from build123d import *

# Parameters (mm, degrees)
BOSS_EXTRUDE1_DEPTH = 4


with BuildPart() as part:
    # Sketch1 → Boss-Extrude1 (new body)
    with BuildSketch(Plane(origin=(0, 0, 0), x_dir=(1, 0, 0), z_dir=(0, 1, 0))):
        with BuildLine():
            ThreePointArc((-5.5, 7.415063509), (-5.646446609, 7.7686169), (-6, 7.915063509))
            Line((-6, 7.915063509), (-9, 7.915063509))
            ThreePointArc((-9, 7.915063509), (-9.353553391, 7.7686169), (-9.5, 7.415063509))
            Line((-9.5, 7.415063509), (-9.5, 1.584936491))
            ThreePointArc((-9.5, 1.584936491), (0, -7.915063509), (9.5, 1.584936491))
            Line((9.5, 1.584936491), (9.5, 7.415063509))
            ThreePointArc((9.5, 7.415063509), (9.353553391, 7.7686169), (9, 7.915063509))
            Line((9, 7.915063509), (6, 7.915063509))
            ThreePointArc((6, 7.915063509), (5.646446609, 7.7686169), (5.5, 7.415063509))
            Line((5.5, 7.415063509), (5.5, 5.915063509))
            ThreePointArc((5.5, 5.915063509), (6.614378278, 3.876224338), (7, 1.584936491))
            ThreePointArc((7, 1.584936491), (0, -5.415063509), (-7, 1.584936491))
            ThreePointArc((-7, 1.584936491), (-6.614378278, 3.876224338), (-5.5, 5.915063509))
            Line((-5.5, 5.915063509), (-5.5, 7.415063509))
        make_face()
    extrude(amount=BOSS_EXTRUDE1_DEPTH)


solid = part.part
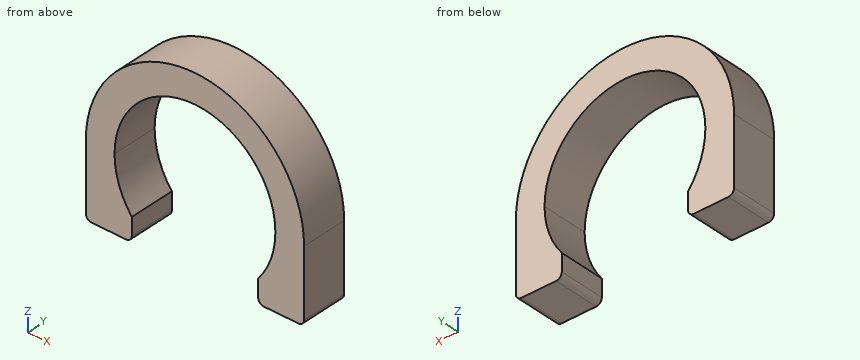
Geometry: final body of the model. Coordinates: model frame, mm. Give positions to 0.01 mm unless a question says otherwise; leave off trailing zeros. Loops run counter-clockwise (first coordinate to the right, second up) from the corner with the lowest first, then second, coordinate; pieces in that order, holes last. Notation, with made-up numbers: M 67,88.5 L 111,88.5 A17 ccw 111,105.5 Z; hole C 70.25,22.25 d9. An arc over 180 degrees is marked long. Put each result on its own line as item: value. Start each with the question number.
1) Ray query, line 1 along X through (y, z) = (2.3, 2.75); line 2 along X through (y, z) = (3.15, 1.75); line 3 along Z through (x, y) = (5.75, 3.25). Return the intervals inside material, ascending.
2) Cut plane A-A (z = -4.5). Output: boundary loops of the cut face in (x, y).
3) Contact query for a flat-ended pin moving along its axis: pin 1 (2 mm diameter, centred on x = 1.5, y = 0.5, fed in from -Z). Output: stop coordinate, or through.
4) Cut plane D-D (z = 1.5). Output: boundary loops of the cut face in (x, y).
5) Cut plane B-B (y = 3.45). Output: boundary loops of the cut face in (x, z).
6) Cut plane C-C (x = 0). Output: boundary loops of the cut face in (y, z), then the cut area to 3 significant figures.
Verdict:
1. line 1: -8.45 to -5.5, 5.5 to 8.45
1. line 2: -8.9 to -6.15, 6.15 to 8.9
1. line 3: -7.85 to -5.58, 2.41 to 5.98
2. outline: M -9.5,0 L -6.36,0 L -6.36,4 L -9.5,4 Z; M 6.36,0 L 9.5,0 L 9.5,4 L 6.36,4 Z
3. pin 1: z = 4.95
4. outline: M -8.99,0 L -6.28,0 L -6.28,4 L -8.99,4 Z; M 6.28,0 L 8.99,0 L 8.99,4 L 6.28,4 Z
5. outline: M -9.5,-7.42 A0.5 ccw -9,-7.92 L -6,-7.92 A0.5 ccw -5.5,-7.42 L -5.5,-5.92 A7 cw long 5.5,-5.92 L 5.5,-7.42 A0.5 ccw 6,-7.92 L 9,-7.92 A0.5 ccw 9.5,-7.42 L 9.5,-1.58 A9.5 ccw -9.5,-1.58 Z
6. outline: M 0,5.42 L 4,5.42 L 4,7.92 L 0,7.92 Z
6. area: 10.0 mm2
